```python
from build123d import *

# Parameters (mm, degrees)
F1_DEPTH     = 44
F0_W         = 27.2
F0_H         = 27.2
F2_DEPTH     = 1
F3_DEPTH     = 37
F4_R         = 4
F4_R_2       = 3
F5_DEPTH     = 25
F6_DEPTH     = 5
F7_R         = 4
F7_R_2       = 3
F8_DEPTH     = 25
F9_DEPTH     = 5
F10_T1_DEPTH = 27.2
F12_DEPTH    = 1


# Not quite as in the source:
# - a fillet or chamfer that OpenCascade refuses, or shapes differently, is made with other operations: its cross-section is extruded or revolved along the edge and cut away or added


with BuildPart() as f1:
    # F0 (on Top) → F1 (new body)
    with BuildSketch(Plane.XY):
        Polygon((49.8359054327, 16.6), (16.6, 16.6), (-16.6, 16.6), (-16.6, 3), (-16.6, 2), (-16.6, -2), (-16.6, -3), (-16.6, -16.6), (16.6, -16.6), (49.8359054327, -16.6), (49.8359054327, -3), (49.8359054327, -2), (49.8359054327, 2), (49.8359054327, 3), align=None)
        Polygon((16.6, -13.6), (13.6, -13.6), (-13.6, -13.6), (-13.6, 13.6), (13.6, 13.6), (16.6, 13.6), (46.1153909564, 13.6), (46.1153909564, -13.6), align=None, mode=Mode.SUBTRACT)
    extrude(amount=F1_DEPTH)

    # F0 (on Top) → F2 (join)
    with BuildSketch(Plane.XY):
        Rectangle(F0_W, F0_H)
        Polygon((16.6, -3), (16.6, -13.6), (46.1153909564, -13.6), (46.1153909564, 13.6), (16.6, 13.6), (16.6, 3), align=None)
    extrude(amount=F2_DEPTH)

    # F0 (on Top) → F3 (join)
    with BuildSketch(Plane.XY):
        Polygon((13.6, 13.6), (13.6, -13.6), (16.6, -13.6), (16.6, -3), (16.6, 3), (16.6, 13.6), align=None)
    extrude(amount=F3_DEPTH)

    # F4 (on face) → F5 (join)
    with BuildSketch(Plane(origin=(-16.6, 0, 0), x_dir=(0, -1, 0), z_dir=(-1, 0, 0))):
        with Locations((0, 7.5)):
            Circle(F4_R)
        with Locations((0, 7.5)):
            Circle(F4_R_2, mode=Mode.SUBTRACT)
    extrude(amount=F5_DEPTH)

    # F6 (cut): a face of the model
    f6_faces = [f1.faces().sort_by_distance(p)[0] for p in [
        (-16.6, 0, 7.5),
    ]]
    extrude(f6_faces, amount=-F6_DEPTH, mode=Mode.SUBTRACT)

    # F7 (on face) → F8 (join)
    with BuildSketch(Plane.YZ.offset(49.8359054327)):
        with Locations((0, 7.5)):
            Circle(F7_R)
        with Locations((0, 7.5)):
            Circle(F7_R_2, mode=Mode.SUBTRACT)
    extrude(amount=F8_DEPTH)

    # F9 (cut): a face of the model
    f9_faces = [f1.faces().sort_by_distance(p)[0] for p in [
        (49.8359054327, 0, 7.5),
    ]]
    extrude(f9_faces, amount=-F9_DEPTH, mode=Mode.SUBTRACT)

    # F10: chamfer of 5 on 1 edges, made by hand

    # F10_s2 → F10_t1 (cut)
    with BuildSketch(Plane.XZ.offset(-13.6)):
        Polygon((16.6, 32), (11.6, 37), (16.6, 37), align=None)
    extrude(amount=F10_T1_DEPTH, mode=Mode.SUBTRACT)

    # F11 (on face) → F12 (join)
    with BuildSketch(Plane.XY.offset(44)):
        with BuildLine():
            ThreePointArc((30.2547216209, 13.6), (31.315381806, 14.0393398209), (31.7547216415, 15.1))
            ThreePointArc((31.7547216415, 15.1), (31.3153818133, 16.1606601718), (30.2547216415, 16.6))
            ThreePointArc((30.2547216415, 16.6), (28.7547216415, 15.1000000103), (30.2547216209, 13.6))
        make_face()
    extrude(amount=F12_DEPTH)


solid = f1.part
```
Work out the finished part from the listing and answer in its coordinate system (mm). A direction names the side the tool comes from. Give positions to 0.01 mm unless a question says otherwise; leave off trailing zeros. Loops run counter-clockwise (first coordinate to the right, second up) from the corner with the lowest first, then second, coordinate; pieces in that order, holes last. Notation, with made-up numbers: M 53.5,-7 L 72.5,-7 A11 ccw 72.5,5 Z; hole C 57.5,-38.75 d7. An arc over 180 degrees is marked long. One line per item, written item: value. Start each with the question number.
1. Find section C-C (z = 25.5). Give the vertices of the cut face in (x, y), and give its area (3 significant figures).
2. Which of the six approach directions +Z, -Z, +X, -X, +Y, -Y give full straight-line access (tool end or side, diameter ignored) to faces 1 (the face through (74.836, -3, 9)), 2 (the face through (-28.925, 0.867, 3.595)), 3 (the face through (15.1, 0.2, 33.5))?
3. Find section B-B (z = 39.5). Give the vertices of the cut face in (x, y).
4. Each of these flat-tipped pins is pushed along its axis until it touches: P1, Ø8, axis at y = 0, z = 7.5, coming from the +X side; P2, Ø8, axis at x = 26.5, y = 4, coming from the +Z side; P3, Ø5.5, axis at y = 0, z = 7.5, coming from the +X side; P4, Ø1.5, axis at y = -13, z = 20, coming from the +X side. Where does it stop, or does it pass through?
5. Find section D-D (x = 53). Give the vertices of the cut face in (y, z), and give its area (3 significant figures).
6. Determine the mould class of faces 4 (the face through (62.161, -0.867, 3.595)), 5 (the face through (22, 13.6, 22)), 6 (the face through (-13.6, 0, 22)), 7 (the face through (17, 16.6, 22)) for opening direction Y: released by +Y, released by -Y, zero draft, split by the parting line, or undercut.
7. Find section A-A (y = 0). Give the vertices of the cut face in (x, z), and give its area (3 significant figures).
8. Find the intervals of material crossed by probe 1 along X at (y, z) = (4, 6); probe 2 along X at (y, z) = (9, 39); probe 3 along Y at (x, z) = (8, 8), in increasing order.
Reported:
1. outline: M -16.6,-16.6 L 49.84,-16.6 L 49.84,16.6 L -16.6,16.6 Z; hole M -13.6,-13.6 L 13.6,-13.6 L 13.6,13.6 L -13.6,13.6 Z; hole M 16.6,-13.6 L 46.12,-13.6 L 46.12,13.6 L 16.6,13.6 Z
1. area: 663 mm²
2. face 1: +Z, -Z, +X, +Y, -Y
2. face 2: -X
2. face 3: +Z
3. outline: M -16.6,-16.6 L 49.84,-16.6 L 49.84,16.6 L -16.6,16.6 Z; hole M -13.6,-13.6 L 46.12,-13.6 L 46.12,13.6 L -13.6,13.6 Z
4. P1: stops at x = 74.84
4. P2: stops at z = 1
4. P3: stops at x = 16.6
4. P4: stops at x = 49.84
5. outline: C 0,7.5 d8; hole C 0,7.5 d6
5. area: 22.0 mm²
6. face 4: split by the parting line
6. face 5: undercut
6. face 6: undercut
6. face 7: released by +Y
7. outline: M -41.6,3.5 L -16.6,3.5 L -16.6,0 L 49.84,0 L 49.84,3.5 L 74.84,3.5 L 74.84,4.5 L 46.12,4.5 L 46.12,1 L 16.6,1 L 16.6,32 L 13.6,35 L 13.6,1 L -13.6,1 L -13.6,4.5 L -41.6,4.5 Z; M -41.6,10.5 L -13.6,10.5 L -13.6,44 L -16.6,44 L -16.6,11.5 L -41.6,11.5 Z; M 46.12,10.5 L 74.84,10.5 L 74.84,11.5 L 49.84,11.5 L 49.84,44 L 46.12,44 Z
7. area: 513 mm²
8. probe 1: x = -16.6 to -13.6, 13.6 to 16.6, 46.12 to 49.84
8. probe 2: x = -16.6 to -13.6, 46.12 to 49.84
8. probe 3: y = -16.6 to -13.6, 13.6 to 16.6
